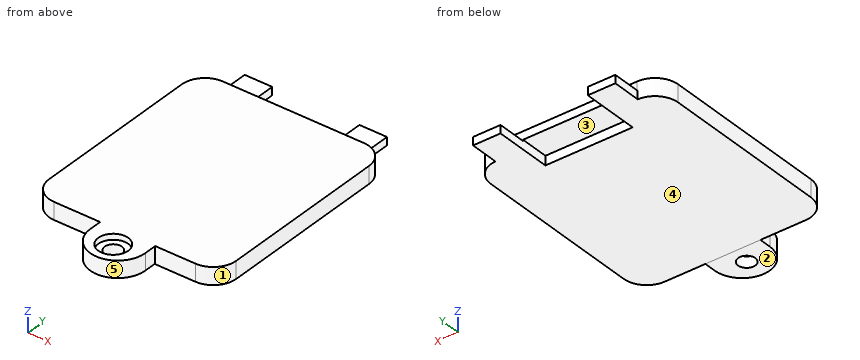
```python
from build123d import *

# Parameters (mm, degrees)
PAD010_DEPTH    = 3
SKETCH044_W     = 15.2
SKETCH044_H     = 5.2
POCKET033_DEPTH = 1.6
SKETCH045_W     = 4.8
SKETCH045_H     = 6
PAD011_DEPTH    = 1.4
PAD012_DEPTH    = 2.9
SKETCH047_R     = 1.5
POCKET034_DEPTH = 5
SKETCH048_R     = 2.6
POCKET035_DEPTH = 1


with BuildPart() as part:
    # Sketch043 → Pad010 (new body)
    with BuildSketch(Plane.XY):
        with BuildLine():
            Line((-48.2, -10.2), (-72.8, -10.2))
            ThreePointArc((-72.8, -10.2), (-75.628427, -11.371573), (-76.8, -14.2))
            Line((-76.8, -14.2), (-76.8, -43.8))
            ThreePointArc((-76.8, -43.8), (-75.628427, -46.628427), (-72.8, -47.8))
            Line((-72.8, -47.8), (-48.2, -47.8))
            ThreePointArc((-48.2, -47.8), (-45.371573, -46.628427), (-44.2, -43.8))
            Line((-44.2, -43.8), (-44.2, -14.2))
            ThreePointArc((-44.2, -14.2), (-45.371573, -11.371573), (-48.2, -10.2))
        make_face()
    extrude(amount=PAD010_DEPTH)

    # Sketch044 (on Face9 of Pad010) → Pocket033 (cut)
    with BuildSketch(Plane(origin=(0, 0, 0), x_dir=(1, 0, 0), z_dir=(0, 0, -1))):
        with Locations((-60.5, 12.6)):
            Rectangle(SKETCH044_W, SKETCH044_H)
    extrude(amount=-POCKET033_DEPTH, mode=Mode.SUBTRACT)

    # Sketch045 (on Face2 of Pocket033) → Pad011 (join)
    with BuildSketch(Plane(origin=(0, 0, 0), x_dir=(1, 0, 0), z_dir=(0, 0, -1))):
        with Locations((-50.5, 8.2)):
            Rectangle(SKETCH045_W, SKETCH045_H)
        with Locations((-70.5, 8.2)):
            Rectangle(SKETCH045_W, SKETCH045_H)
    extrude(amount=-PAD011_DEPTH)

    # Sketch046 (on Face10 of Pad011) → Pad012 (join)
    with BuildSketch(Plane.XY.offset(3)):
        with BuildLine():
            ThreePointArc((-64.8, -50), (-60, -54.8), (-55.2, -50))
            Line((-55.2, -47.8), (-55.2, -50))
            Line((-64.8, -47.8), (-55.2, -47.8))
            Line((-64.8, -50), (-64.8, -47.8))
        make_face()
    extrude(amount=-PAD012_DEPTH)

    # Sketch047 (on Face24 of Pad012) → Pocket034 (cut)
    with BuildSketch(Plane.XY.offset(3)):
        with Locations((-60, -51)):
            Circle(SKETCH047_R)
    extrude(amount=-POCKET034_DEPTH, mode=Mode.SUBTRACT)

    # Sketch048 (on Face5 of Pocket034) → Pocket035 (cut)
    with BuildSketch(Plane.XY.offset(3)):
        with Locations((-60, -51)):
            Circle(SKETCH048_R)
    extrude(amount=-POCKET035_DEPTH, mode=Mode.SUBTRACT)


with BuildPart() as part_1:
    # Body002 placement: moved
    add(part.part.moved(Location((0, 0, 35))))


solid = part_1.part
```
Read the model definition and answer for the solid it produces. Units are mm, in the model's axes. Face numbers are marked on the shaded views. A direction names the side the tool comes from. Give positions to 0.01 mm unless a question says otherwise; leave off trailing zeros. Loops run counter-clockwise (first coordinate to the right, second up) from the corner with the lowest first, then second, coordinate; pieces in that order, holes last.
Item 1: For the marked faces 1 and 2, determine the directions among +Z, -Z, +X, -X, +Y, -Y from which every point of the face is accessible in a straight line to the end or side of a thin tool.
Item 2: The part is cut by section C-C (x = -69). Write down the section's boundary in (y, z), and give its area (3 significant figures).
Item 3: The mould has two halves that part along X. Classify the marked faces 3, 4 and 5: released by +X, released by -X, zero draft, split by the parting line, or undercut.
Item 4: Find the intervals of material crossed by line 1 along X through (y, z) = (-10, 35.8); line 2 along Y through (x, z) = (-60, 37.25); line 3 along Y through (x, z) = (-69.5, 35.6), in increasing order.
Item 5: The part is cut by section B-B (y = -51). Write down the section's boundary in (x, z).
Item 6: The part is cut by section A-A (x = -60). Write down the section's boundary in (y, z), and give its area (3 significant figures).
Item 7: Each of these flat-tipped pins is pushed along its axis until it touches: pin 1 Ø4 at (x, y) = (-71, -8) entering from +Z; pin 2 Ø1.3 at (y, z) = (-11, 35.5) entering from -X; pin 3 Ø1.1 at (y, z) = (-7.5, 35.5) entering from +X. Where does it stop, or does it pass through?
Taken from the geometry:
1. face 1: +Z, -Z, +X, -Y
1. face 2: -Z, +X, -X, -Y
2. outline: (-47.8, 35) - (-5.2, 35) - (-5.2, 36.4) - (-10.2, 36.4) - (-10.2, 38) - (-47.8, 38) - close
2. area: 120 mm2
3. face 3: undercut
3. face 4: zero draft
3. face 5: split by the parting line
4. line 1: x = -72.9 to -68.1, -52.9 to -48.1
4. line 2: y = -54.8 to -53.6, -48.4 to -10.2
4. line 3: y = -47.8 to -5.2
5. outline: (-64.69, 35.1) - (-61.5, 35.1) - (-61.5, 37) - (-62.6, 37) - (-62.6, 38) - (-64.69, 38) - close; (-58.5, 35.1) - (-55.31, 35.1) - (-55.31, 38) - (-57.4, 38) - (-57.4, 37) - (-58.5, 37) - close
6. outline: (-54.8, 35.1) - (-52.5, 35.1) - (-52.5, 37) - (-53.6, 37) - (-53.6, 38) - (-54.8, 38) - close; (-49.5, 35.1) - (-47.8, 35.1) - (-47.8, 35) - (-15.2, 35) - (-15.2, 36.6) - (-10.2, 36.6) - (-10.2, 38) - (-48.4, 38) - (-48.4, 37) - (-49.5, 37) - close
6. area: 114 mm2
7. pin 1: stops at z = 36.4
7. pin 2: stops at x = -75.88
7. pin 3: stops at x = -48.1
